```python
from build123d import *

# Parameters (mm, degrees)
BOSS_EXTRUDE1_DEPTH = 8.2


with BuildPart() as part:
    # Sketch1 → Boss-Extrude1 (new body)
    with BuildSketch(Plane.XY):
        with BuildLine():
            Line((5.002809822, -2.4), (-27, -2.4))
            Line((-27, -2.4), (-27, 5.24803322))
            Line((-27, 5.24803322), (-26.145643924, 5.24803322))
            ThreePointArc((-26.145643924, 5.24803322), (-23.75, 5.74803322), (-26.145643924, 6.24803322))
            Line((-26.145643924, 6.24803322), (-27, 6.24803322))
            Line((-27, 6.24803322), (-27, 13.9))
            Line((-27, 13.9), (5.002809822, 13.9))
            Line((5.002809822, 13.9), (5.002809822, 6.24803322))
            Line((5.002809822, 6.24803322), (4.148453745, 6.24803322))
            ThreePointArc((4.148453745, 6.24803322), (1.752809822, 5.74803322), (4.148453745, 5.24803322))
            Line((4.148453745, 5.24803322), (5.002809822, 5.24803322))
            Line((5.002809822, 5.24803322), (5.002809822, -2.4))
        make_face()
        with BuildLine():
            Line((-10.5, 8.65), (-10.826670764, 8.65))
            ThreePointArc((-10.826670764, 8.65), (-22.4, 5.75), (-10.826670764, 2.85))
            Line((-10.826670764, 2.85), (-10.5, 2.85))
            ThreePointArc((-10.5, 2.85), (-7.6, 5.75), (-10.5, 8.65))
        make_face(mode=Mode.SUBTRACT)
    extrude(amount=BOSS_EXTRUDE1_DEPTH)


solid = part.part
```
The model under review builds one solid part; all positions refer to its coordinate system, in mm. A direction names the side the tool comes from. Round coordinates to 2 decimals unless told otherwise and drop trailing zeros. Order: outer loops, then holes, each group sorted by start corner. A loop starts at its lowest first (then second) coordinate and runs counter-clockwise, first axis right, second up. Notation, with made-up numbers: (80.5, 26.25) -> (139.5, 26.25) arc R25 cw to (139.5, 51.25) -> close; hole circle Ø1 at (9, 80.5). An arc over 180 degrees is marked (long way). One line per item, written item: value. Start each with the question number.
Q1. Take a section at A-A (x = -25). Write out the cut boundary in (y, z), and give its area (3 significant figures).
Q2. Machinability: for faces 1 (the face through (-26.6, 6.248, 4)), 2 (the face through (4.6, 6.248, 4)), 3 (the face through (-7.6, 5.7, 4)), which of the approach directions +Z, -Z, +X, -X, +Y, -Y give a long, thin tool a straight path to every point of the face, cutting with its end or side? Answer none if there is none.
Q3. Take a section at B-B (y = 5.75). Write out the cut boundary in (x, z), and give its area (3 significant figures).
Q4. Take a section at C-C (z = 3.5). Write out the cut boundary in (x, y).
Q5. Mouldability with a two-part tool opening along Y and no side actions: class faces 4 (the face through (-11, -2.4, 4)), 5 (the face through (-22.396, 5.978, 4.043)), 6 (the face through (-11, 13.9, 4)), 7 (the face through (-26.6, 5.248, 4)) as released by +Y, released by -Y, zero draft, split by the parting line, or undercut.
Q6. Wall thickness on line 1 (Y direction, x = -16.25, z = 3.25); line 2 (Y direction, x = -25, z = 6); line 3 (X direction, y = 6.75, z = 2.5): over which ranges is each line inside the solid? List them lowest first.
Reported:
1. outline: (-2.4, 0) -> (4.5, 0) -> (4.5, 8.2) -> (-2.4, 8.2) -> close; (7, 0) -> (13.9, 0) -> (13.9, 8.2) -> (7, 8.2) -> close
1. area: 113 mm2
2. face 1: +Z, -Z, -X
2. face 2: +Z, -Z, +X
2. face 3: +Z, -Z
3. outline: (-23.75, 0) -> (-22.4, 0) -> (-22.4, 8.2) -> (-23.75, 8.2) -> close; (-7.6, 0) -> (1.75, 0) -> (1.75, 8.2) -> (-7.6, 8.2) -> close
3. area: 87.8 mm2
4. outline: (-27, -2.4) -> (5, -2.4) -> (5, 5.25) -> (4.15, 5.25) arc R1.25 cw (long way) to (4.15, 6.25) -> (5, 6.25) -> (5, 13.9) -> (-27, 13.9) -> (-27, 6.25) -> (-26.15, 6.25) arc R1.25 cw (long way) to (-26.15, 5.25) -> (-27, 5.25) -> close; hole (-10.83, 2.85) -> (-10.5, 2.85) arc R2.9 ccw to (-10.5, 8.65) -> (-10.83, 8.65) arc R6.15 ccw (long way) to start
5. face 4: released by -Y
5. face 5: undercut
5. face 6: released by +Y
5. face 7: undercut
6. line 1: y = -2.4 to -0.4, 11.9 to 13.9
6. line 2: y = -2.4 to 4.5, 7 to 13.9
6. line 3: x = -27 to -25.75, -24.25 to -22.32, -7.78 to 2.26, 3.75 to 5
